```python
from build123d import *

# Parameters (mm, degrees)
F0_W     = 48.26
F0_H     = 48.26
F1_DEPTH = 3.175
F0_W_2   = 53.975
F0_H_2   = 53.975
F2_DEPTH = 25.4
F4_DEPTH = 53.975
F5_W     = 15.875
F5_H     = 3.175
F6_DEPTH = 63.5


with BuildPart() as f1:
    # F0 (on Top) → F1 (new body)
    with BuildSketch(Plane.XY):
        Rectangle(F0_W, F0_H)
    extrude(amount=F1_DEPTH)

    # F0 (on Top) → F2 (join)
    with BuildSketch(Plane.XY):
        Rectangle(F0_W_2, F0_H_2)
        Rectangle(F0_W, F0_H, mode=Mode.SUBTRACT)
    extrude(amount=F2_DEPTH)

    # F3 (on face) → F4 (join)
    with BuildSketch(Plane.XZ.offset(26.9875)):
        with BuildLine():
            Line((26.9875, 0), (-26.9875, 0))
            Line((-26.9875, 0), (-26.9875, -25.4))
            Line((-26.9875, -25.4), (-23.8125, -25.4))
            ThreePointArc((-23.8125, -25.4), (-0.052452, -3.175), (23.707596, -25.4))
            Line((23.707596, -25.4), (26.882596, -25.4))
            Line((26.882596, -25.4), (26.9875, 0))
        make_face()
    extrude(amount=-F4_DEPTH)

    # F5 (on face) → F6 (cut)
    with BuildSketch(Plane(origin=(26.98704, 0, -0.111459), x_dir=(0, 1, 0), z_dir=(0.999991, 0, -0.00413))):
        with Locations((-15.875, -20.73563)):
            Rectangle(F5_W, F5_H)
        with Locations((15.875, -20.73563)):
            Rectangle(F5_W, F5_H)
    extrude(amount=-F6_DEPTH, mode=Mode.SUBTRACT)


solid = f1.part
```
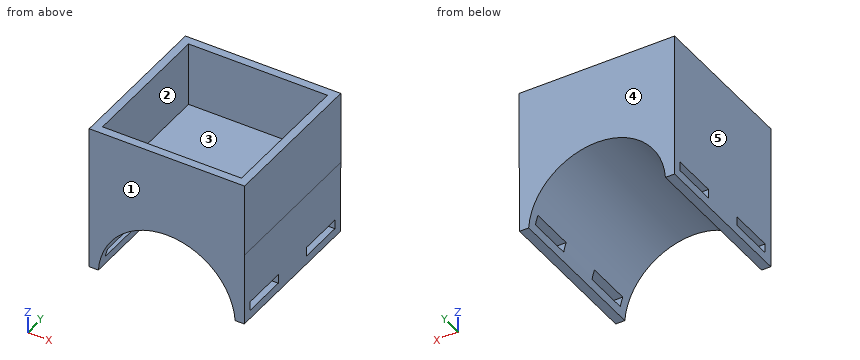
Work out the finished part from the listing and answer in its coordinate system (mm). Face numbers are marked on the shaded views. A direction names the side the tool comes from. Give positions to 0.01 mm unless a question says otherwise; leave off trailing zeros. Order: outer loops, then holes, each group sorted by start corner. A loop starts at its lowest first (then second) coordinate and runs counter-clockwise, first axis right, second up. Notation, with made-up numbers: M 69,-35.75 L 76,-35.75 A5 cw 76,-28.75 Z; hole C -16,29.25 d1. An arc over 180 degrees is marked long. Return JSON: item names as keys, results as strings.
1) Section A-A, the plane y = 21 is taken. Write down the section's boundary in (x, z) (1 decimal), plus the area to 3 significant figures.
Resolved:
{"outline": "M -27,-25.4 L -23.8,-25.4 A23.8 cw -23.4,-22.2 L -27,-22.2 Z; M -27,-19 L -22.5,-19.1 A23.8 cw 22.5,-19.2 L 26.9,-19.3 L 27,0 L 27,25.4 L 24.1,25.4 L 24.1,3.2 L -24.1,3.2 L -24.1,25.4 L -27,25.4 Z; M 23.3,-22.4 A23.8 cw 23.7,-25.4 L 26.9,-25.4 L 26.9,-22.4 Z", "area": "828 mm^2"}
2) A tool of negligible diameter and unlimited length cuts with its end or side. For the marked faces 1 and 2, from which of +Z, -Z, +X, -X, +Y, -Y can it reach the whole face along a straight path? Write none if from no direction.
Resolved:
{"face 1": "+Z, -Z, +X, -X, -Y", "face 2": "+Z"}
3) Each of these flat-tipped pins is pushed along its axis until it touches: pin 1 (12 mm diameter, centred on x = 3, y = 14.5, fed in from -Z); pin 2 (10 mm diameter, centred on x = -12.5, y = -8, fed in from -Z); pin 3 (8 mm diameter, centred on y = -6, z = -13, fed in from +X). Where does it stop, or does it pass through?
Resolved:
{"pin 1": "z = -4.96", "pin 2": "z = -10.78", "pin 3": "x = 26.95"}
4) Section D-D, the plane z = -5.5 is taken. Write down the section's boundary in (x, y), plus the area to 3 significant figures.
Resolved:
{"outline": "M -26.99,-26.99 L -10.32,-26.99 L -10.32,26.99 L -26.99,26.99 Z; M 10.21,-26.99 L 26.96,-26.99 L 26.96,26.99 L 10.21,26.99 Z", "area": "1,800 mm^2"}
5) For a pull along X with two mould halves and no side action, classify the marked faces 3, 4 and 5 as +X half, -X half, draft (parallel to the pull), parting line (faces both ways), or undercut.
Resolved:
{"face 3": "undercut", "face 4": "draft", "face 5": "-X half"}
6) Section B-B, the plane y = 4 is taken. Write down the section's boundary in (x, z) (1 decimal), plus the area to 3 significant figures.
Resolved:
{"outline": "M -27,-25.4 L -23.8,-25.4 A23.8 cw 23.7,-25.4 L 26.9,-25.4 L 27,0 L 27,25.4 L 24.1,25.4 L 24.1,3.2 L -24.1,3.2 L -24.1,25.4 L -27,25.4 Z", "area": "853 mm^2"}
7) Straight lines are drawn through the part: line 1 along Y through (x, z) = (8, 13.5); line 2 along X through (y, z) = (-4, -16.5). For each, find the intervals that lie inside material, in ascending order. Write a range as [from, to].
Resolved:
{"line 1": "[-26.99, -24.13], [24.13, 26.99]", "line 2": "[-26.99, -21.43], [21.33, 26.92]"}
8) Section C-C, the plane z = 12 is taken. Write down the section's boundary in (x, y), plus the area to 3 significant figures.
Resolved:
{"outline": "M -26.99,-26.99 L 26.99,-26.99 L 26.99,26.99 L -26.99,26.99 Z; hole M -24.13,-24.13 L 24.13,-24.13 L 24.13,24.13 L -24.13,24.13 Z", "area": "584 mm^2"}
